Verification items for this drawing (mm, ordinates from the low corner). A direction names the side the tool comes from. Give positions to 0.01 mm unless a question says otherwise; leave off trailing zeros. Loops run counter-clockwise (first coordinate to the right, second up) from the corner with the lowest first, then second, coordinate; pieces in that order, holes last. Notation, with made-up numbers: M 2,51.25 L 11,51.25 A22 ccw 11,84.25 Z; hole C 58,-7.75 d11. An arc over 180 degrees is marked long. Answer in a Markdown table with one row per item.
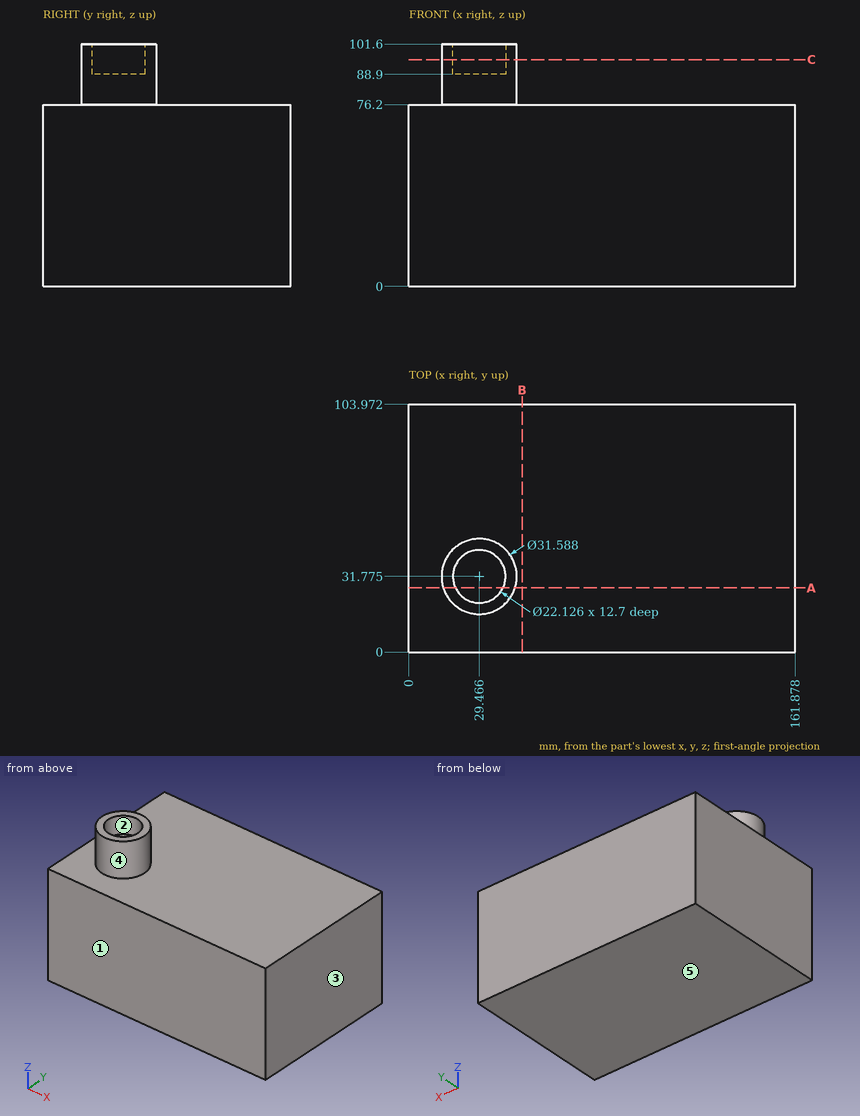
Item 1: Go/stop test with flat-tipped pins: pin 1 (2 mm diameter, centred on x = 111, y = 77, fed in from +Z); pin 2 (13.5 mm diameter, centred on x = 29.47, y = 31.78, fed in from +Z). Record where each tip stops, or that it passes through.
Reported:
| item | result |
|---|---|
| pin 1 | stops at z = 76.2 |
| pin 2 | stops at z = 88.9 |
Item 2: Sectioned sample at B-B (x = 47.5). Record the cut outline in (y, z).
Reported:
| item | result |
|---|---|
| outline | M 0,0 L 103.97,0 L 103.97,76.2 L 0,76.2 Z |
Item 3: Sectioned sample at C-C (z = 95). Record the cut outline in (x, y) (1 decimal), and give its area (3 significant figures).
Reported:
| item | result |
|---|---|
| outline | C 29.5,31.8 d31.6; hole C 29.5,31.8 d22.1 |
| area | 399 mm^2 |
Item 4: Sectioned sample at A-A (y = 27). Record the cut outline in (x, z) (1 decimal), and give its area (3 significant figures).
Reported:
| item | result |
|---|---|
| outline | M 0,0 L 161.9,0 L 161.9,76.2 L 44.5,76.2 L 44.5,101.6 L 39.4,101.6 L 39.4,88.9 L 19.5,88.9 L 19.5,101.6 L 14.4,101.6 L 14.4,76.2 L 0,76.2 Z |
| area | 12,800 mm^2 |
Item 5: Tool access check on the marked faces 4 and 5. Record the directions out of +Z, -Z, +X, -X, +Y, -Y that give a thin tool (end or side, any length) a straight path to the whole face; none if there is none.
Reported:
| item | result |
|---|---|
| face 4 | +Z |
| face 5 | -Z, +X, -X, +Y, -Y |
Item 6: Release check for a two-part mould opening along Y. For the marked faces 1, 2 and 3 record: released by +Y, released by -Y, zero draft, split by the parting line, or undercut.
Reported:
| item | result |
|---|---|
| face 1 | released by -Y |
| face 2 | undercut |
| face 3 | zero draft |
Item 7: Scan lines: L1, parallel to Z at x = 43.5, y = 76; L2, parallel to X at y = 42.5, z = 88.5 (1 decimal); L3, parallel to X at y = 17.5, z = 90 (1 decimal). Record each from-to range of solid material in increasing order. Write a range as [from, to].
Reported:
| item | result |
|---|---|
| L1 | z = [0, 76.2] |
| L2 | x = [17.9, 41.1] |
| L3 | x = [22.7, 36.2] |
